Check sheet for the modelled part. Datum: model origin and axes. Units: mm. A direction names the side the tool comes from. Coordinates: 2 decimals unless noted, no trailing zeros. Write each loop counter-clockwise with the first axis right and the second up, starting at its lowest first coordinate (ties: lowest second). Pieces come first, ordered by that corner, then holes. Notation, with made-up numbers: M 60.5,14 L 65.5,14 A13 ccw 65.5,25 Z; hole C 35.5,-36.75 d10. An arc over 180 degrees is marked long. Answer as CSV lines item,"result". Start each with the question number.
1) Section check C-C (y = 37). Record the cut outline in (x, z).
2) Go/stop test with flat-tipped pins: pin 1 Ø12 at (y, z) = (86.5, 5.5) entering from +X; pin 2 Ø1.5 at (x, z) = (135.5, -3.5) entering from +Y; pin 3 Ø1.5 at (y, z) = (103, -3) entering from +X. Record where each tip stops, or that it passes through.
3) Section check A-A (z = -1.5). Record the cut outline in (x, y).
4) Draft check along Y on faces 3 (the flat face through (87.52, 120.25, 0.13)), 4 (the flat face through (-13, 20, 1)), 5 (the flat face through (185, 206, 1)). Enter one of: +Y half, -Y half, draft (parallel to the pull), parting line (faces both ways), or undercut.
5) Section check B-B (x = 136). Record the cut outline in (y, z).
6) Access from +Z, -Z, +X, -X, +Y, -Y to the whole of each face (thin tool, end or side, straight path). Record for faces 1 (the flat face through (90, 117, 9)), 2 (the flat face through (91, 111, 0)).
7) Material ranges on L1, parallel to Z at x = 16, y = 44.5; L2, parallel to Y at x = 30.5, z = 5.5; L3, parallel to X at y = 206, z = -4, recorded low to high. Write a range as [from, to].
from build123d import *

# Parameters (mm, degrees)
EXTRUDE_1_DEPTH          = 10
CUT_EXTRUDE_1_DEPTH      = 273.883551892
CUT_EXTRUDE_1_DEPTH_BACK = 273.883551892
SKETCH_2_W               = 18
SKETCH_2_H               = 8
SKETCH_3_R               = 1.6
CUT_EXTRUDE_2_DEPTH      = 286.946556009


with BuildPart() as part:
    # 草图1 → 凸台-拉伸1 (new, symmetric)
    with BuildSketch(Plane.XY):
        Polygon((0, 20), (185, 205), (185, 219.142135624), (-14.142135624, 20), align=None)
    extrude(amount=EXTRUDE_1_DEPTH, both=True)

    # 草图2 → 切除-拉伸1 (cut, two sides: drawn at the far end of the back side and taken through both)
    with BuildSketch(Plane(origin=(10, 10, 0), x_dir=(0, 0, -1), z_dir=(-0.7071067811865462, -0.7071067811865489, 0)).offset(-CUT_EXTRUDE_1_DEPTH_BACK)):
        with Locations((0, -19.142135624)):
            Rectangle(SKETCH_2_W, SKETCH_2_H)
    extrude(amount=CUT_EXTRUDE_1_DEPTH + CUT_EXTRUDE_1_DEPTH_BACK, mode=Mode.SUBTRACT)

    # 草图3 → 切除-拉伸2 (cut, through all)
    with BuildSketch(Plane(origin=(-17.071067812, 17.071067812, 0), x_dir=(0.7071067811865462, 0.707106781186549, 0), z_dir=(-0.707106781186549, 0.7071067811865462, 0))):
        with Locations(Location((247.771644663, 6, 0), (0, 0, 180))):
            Circle(SKETCH_3_R)
        with Locations(Location((247.771644663, -6, 0), (0, 0, 180))):
            Circle(SKETCH_3_R)
    extrude(amount=-CUT_EXTRUDE_2_DEPTH, mode=Mode.SUBTRACT)


solid = part.part
Results found:
1,outline,"M 2.86,-10 L 17,-10 L 17,10 L 2.86,10 Z; hole M 4.27,-9 L 15.59,-9 L 15.59,9 L 4.27,9 Z"
2,pin 1,"stops at x = 72.5"
2,pin 2,"stops at y = 170.39"
2,pin 3,"stops at x = 83.75"
3,outline,"M -14.14,20 L -12.73,20 L 185,217.73 L 185,219.14 Z; M -1.41,20 L 0,20 L 185,205 L 185,206.41 Z"
4,face 3,"undercut"
4,face 4,"-Y half"
4,face 5,"draft"
5,outline,"M 156,-10 L 170.14,-10 L 170.14,10 L 156,10 Z; hole M 157.41,-9 L 168.73,-9 L 168.73,9 L 157.41,9 Z"
6,face 1,"none"
6,face 2,"+Z, -Z, +X, -Y"
7,L1,"z = [-10, -9], [9, 10]"
7,L2,"y = [50.5, 51.91], [63.23, 64.64]"
7,L3,"x = [171.86, 173.27], [184.59, 185]"
